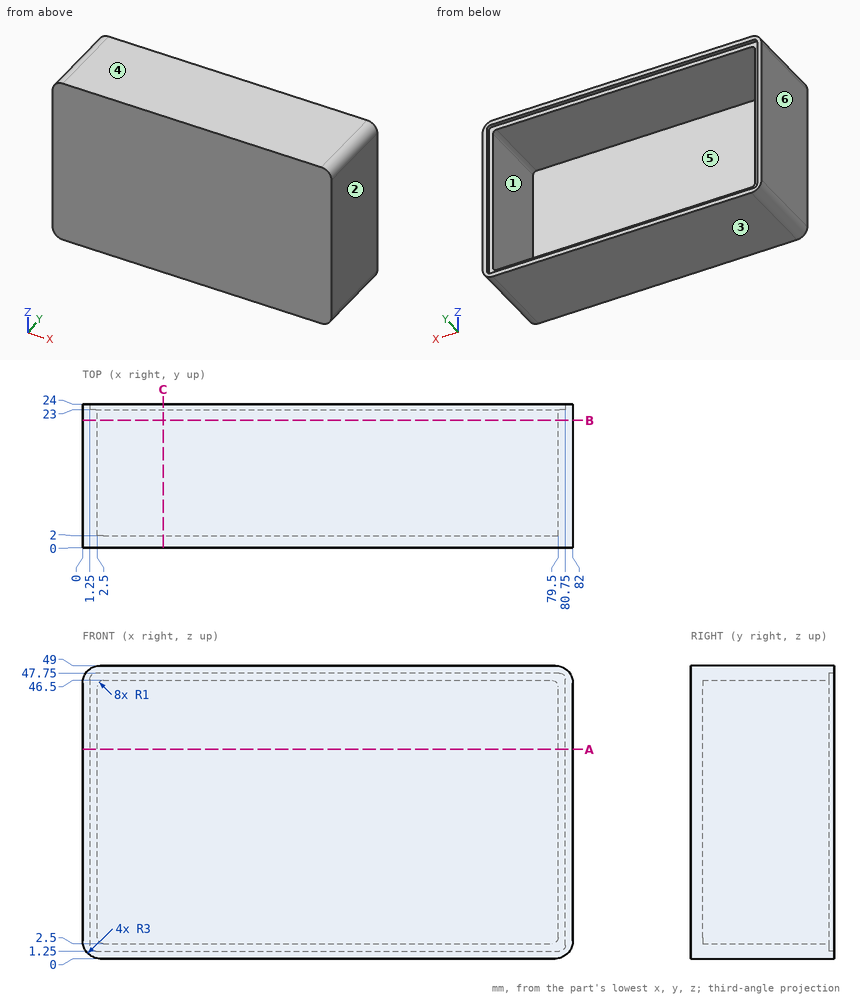
Here's the drawing with two shaded views (mm, measured from the low corner). I have some questions. A direction names the side the tool comes from. Give positions to 0.01 mm unless a question says otherwise; leave off trailing zeros. Loops run counter-clockwise (first coordinate to the right, second up) from the corner with the lowest first, then second, coordinate; pieces in that order, holes last. Notation, with made-up numbers: M 46,-35.75 L 70,-35.75 A20 cw 70,-18.75 Z; hole C 61,-34 d8. An arc over 180 degrees is marked long. One line per item, written item: value.
(1) Will this pin go through, and if not, where does the flat tip stop? pin 1 (4 mm diameter, centred on x = 49.5, z = 41.5, fed in from +Y).
Returned:
pin 1: y = 2
(2) Suppose I cut it at B-B on y = 21.25. List the corners of the cut face in (x, z) for me, plus the area to 3 significant figures.
Returned:
outline: M 0,3 A3 ccw 3,0 L 79,0 A3 ccw 82,3 L 82,46 A3 ccw 79,49 L 3,49 A3 ccw 0,46 Z; hole M 2.5,3.5 A1 ccw 3.5,2.5 L 78.5,2.5 A1 ccw 79.5,3.5 L 79.5,45.5 A1 ccw 78.5,46.5 L 3.5,46.5 A1 ccw 2.5,45.5 Z
area: 623 mm^2
(3) I need wall thicknesses on line 1 (Z direction, x = 76.5, y = 9.75); line 2 (X direction, y = 22.25, z = 37); line 3 (Y direction, x = 33, z = 33). Which ranges of each line are inside material? Lowest first, please.
Returned:
line 1: 0 to 2.5, 46.5 to 49
line 2: 0 to 2.5, 79.5 to 82
line 3: 0 to 2
(4) Which directions (+Z, -Z, +X, -X, +Y, -Y) give clear straight access to the entire face, cutting with the end or side of a thin tool? Please do the marked faces 1 and 2.
Returned:
face 1: +Y
face 2: +Z, -Z, +X, +Y, -Y
(5) We'd pull the mould along Z, two halves only. Please class the marked faces 3, 4, 5 and 6: released by +Z, released by -Z, zero draft, split by the parting line, or undercut.
Returned:
face 3: released by -Z
face 4: released by +Z
face 5: undercut
face 6: zero draft
(6) Suppose I cut it at C-C on x = 13.5. List the corners of the cut face in (y, z) for me, plus the area to 4 significant figures.
Returned:
outline: M 0,0 L 24,0 L 24,1.25 L 23,1.25 L 23,2.5 L 2,2.5 L 2,46.5 L 23,46.5 L 23,47.75 L 24,47.75 L 24,49 L 0,49 Z
area: 205.5 mm^2
(7) Suppose I cut it at A-A on z = 35. List the corners of the cut face in (x, y) for me.
Returned:
outline: M 0,0 L 82,0 L 82,24 L 80.75,24 L 80.75,23 L 79.5,23 L 79.5,2 L 2.5,2 L 2.5,23 L 1.25,23 L 1.25,24 L 0,24 Z
